The listing builds one solid part. Answer for the finished solid, in the listing's coordinates (mm). Face numbers are marked on the shaded views. A direction names the side the tool comes from. Round coordinates to 2 decimals unless told otherwise and drop trailing zeros. Loops run counter-clockwise (first coordinate to the right, second up) from the corner with the lowest first, then second, coordinate; pieces in that order, holes last. Notation, with made-up numbers: M 73.5,11.25 L 104.5,11.25 A21 ccw 104.5,48.25 Z; hole C -12.75,-29 d2. An arc over 180 degrees is marked long. Answer as a JSON object with one key per item and string values.
```python
from build123d import *

# Parameters (mm, degrees)
F0_W     = 7.62
F0_H     = 34.036
F0_W_2   = 5.207
F0_H_2   = 30.48
F1_DEPTH = 1.016
F2_SIZE2 = 0.2041772846
F2_SIZE  = 0.762
F3_R     = 0.254
F4_R     = 3.048
F5_W     = 5.08
F5_H     = 34.036
F6_DEPTH = 3.048


with BuildPart() as f1:
    # F0 (on Top) → F1 (new body)
    with BuildSketch(Plane.XY):
        with Locations((3.81, 17.018)):
            Rectangle(F0_W, F0_H)
        with Locations((4.3815, 17.018)):
            Rectangle(F0_W_2, F0_H_2, mode=Mode.SUBTRACT)
    extrude(amount=F1_DEPTH)

    # F2
    f2_edges = [f1.edges().sort_by_distance(p)[0] for p in [
        (0, 17.018, 0),
    ]]
    f2_side = f1.faces().sort_by_distance((0.348786, 17.018, 0))[0]
    chamfer(f2_edges, length=F2_SIZE, length2=F2_SIZE2, reference=f2_side)

    # F3
    f3_edges = [f1.edges().sort_by_distance(p)[0] for p in [
        (0, 17.018, 0.204177),
    ]]
    fillet(f3_edges, radius=F3_R)

    # F4
    f4_edges = [f1.edges().sort_by_distance(p)[0] for p in [
        (0.762, 17.018, 0),
    ]]
    fillet(f4_edges, radius=F4_R)

    # F5 (on Top) → F6 (join)
    with BuildSketch(Plane.XY):
        with Locations((10.16, 17.018)):
            Rectangle(F5_W, F5_H)
    extrude(amount=F6_DEPTH)


solid = f1.part
```
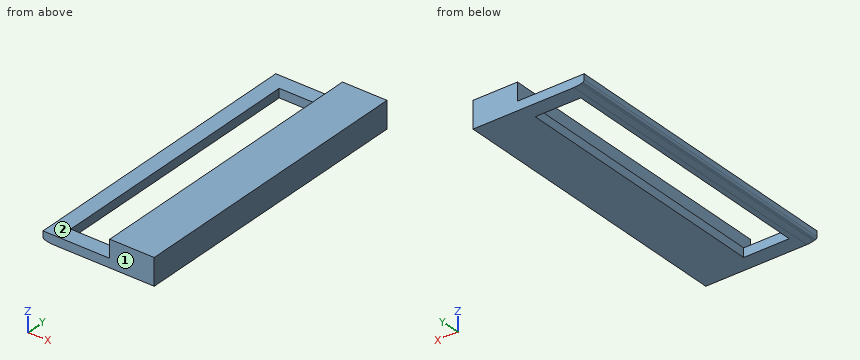
Item 1: The part is cut by section B-B (x = 5.5). Give the vertices of the cut face in (y, z), then the cut area to 3 significant figures.
Values follow:
{"outline": "M 0,0 L 1.78,0 L 1.78,1.02 L 0,1.02 Z; M 32.26,0 L 34.04,0 L 34.04,1.02 L 32.26,1.02 Z", "area": "3.61 mm^2"}
Item 2: The part is cut by section C-C (z = 2.2). Give the vertices of the cut face in (x, y).
Values follow:
{"outline": "M 7.62,0 L 12.7,0 L 12.7,34.04 L 7.62,34.04 Z"}
Item 3: Straight lines are drawn through the part: line 1 (X direction, y = 10, z = 0.85) (3 decimals); line 2 (X direction, y = 5.5, z = 0.2) (3 decimals); line 3 (X direction, y = 11, z = 2.2). For each, find the intervals that lie inside material, in ascending order.
Values follow:
{"line 1": "0 to 1.778, 6.985 to 12.7", "line 2": "0.096 to 1.778, 6.985 to 12.7", "line 3": "7.62 to 12.7"}
Item 4: Which of the six approach directions +Z, -Z, +X, -X, +Y, -Y give full straight-line access (tool end or side, diameter ignored) to the marked faces 1 and 2?
Values follow:
{"face 1": "+Z, -Z, +X, -X, -Y", "face 2": "+Z, -X, +Y, -Y"}
Item 5: The part is cut by section A-A (y = 4.5). Give the vertices of the cut face in (x, z) (3 decimals), then the cut area to 3 significant figures.
Values follow:
{"outline": "M 0,0.399 A0.254 ccw 0.188,0.154 L 0.374,0.104 A3.048 ccw 1.163,0 L 1.778,0 L 1.778,1.016 L 0,1.016 Z; M 6.985,0 L 12.7,0 L 12.7,3.048 L 7.62,3.048 L 7.62,1.016 L 6.985,1.016 Z", "area": "17.8 mm^2"}
Item 6: Flat-ended cylindrical pins translate along their axes: P1, Ø1.5, axis at y = 27.5, z = 2.5, coming from the -X side; P2, Ø4, axis at x = 2, y = 28.5, coming from the +Z side. Find the tip coordinate at first contact, or state that the pin passes through.
Values follow:
{"P1": "x = 7.62", "P2": "z = 1.02"}
